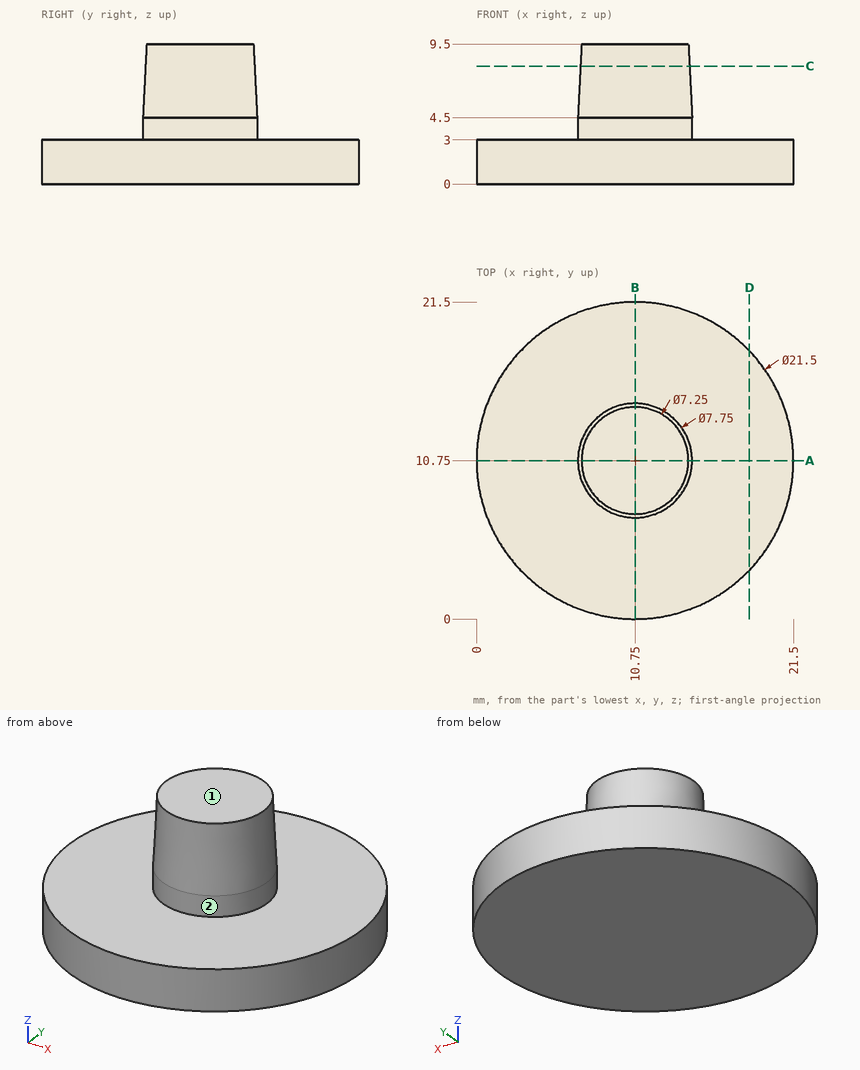
Could you check a few things on this drawing? It's one solid part, dimensions in mm from its lowest x, y, z. A direction names the side the tool comes from. Give positions to 0.01 mm unless a question says otherwise; leave off trailing zeros. Write each loop counter-clockwise with the first axis right and the second up, starting at its lowest first coordinate (ties: lowest second). Pieces come first, ordered by that corner, then holes. Notation, with made-up numbers: M 59.25,89 L 106.25,89 A13 cw 106.25,112 Z; hole C 12.5,83 d3. An arc over 180 degrees is marked long. Put each result on its own line as item: value. Start each with the question number.
Item 1: I need wall thicknesses on L1, parallel to Z at x = 9.25, y = 19; L2, parallel to X at y = 13, z = 1; L3, parallel to X at y = 8, z = 4.25. Which ranges of each line are inside material? Lowest first, please. Write a range as from..to.
Item 2: If we section it at A-A, the plane y = 10.75: Write out the boundary of the cut face in (x, z) (3 decimals).
Item 3: Will these pins go through, and if not, where does the flat tip stop? pin 1 (4 mm diameter, centred on x = 3, z = 4.5, fed in from +Y); pin 2 (1 mm diameter, centred on x = 7, z = 7.5, fed in from -Y); pin 3 (5 mm diameter, centred on x = 11, z = 6.5, fed in from -Y) (3 decimals).
Item 4: If we section it at C-C, the plane z = 8: Write out the boundary of the cut face in (x, y).
Item 5: If we section it at D-D, the plane x = 18.5: Write out the boundary of the cut face in (y, z).
Item 6: On a 3-axis mill with a long thin cutter (end or side, diameter ignored), from which of +Z, -Z, +X, -X, +Y, -Y can I reach the whole of each face in a straight line? I mean the marked faces 1 and 2. Say none if no direction works.
Values:
1. L1: 0..3
1. L2: 0.24..21.26
1. L3: 8.02..13.48
2. outline: M 0,0 L 21.5,0 L 21.5,3 L 14.625,3 L 14.625,4.5 L 14.375,9.5 L 7.125,9.5 L 6.875,4.5 L 6.875,3 L 0,3 Z
3. pin 1: y = 19.37
3. pin 2: y = 8.93
3. pin 3: y = 6.875
4. outline: C 10.75,10.75 d7.4
5. outline: M 3.3,0 L 18.2,0 L 18.2,3 L 3.3,3 Z
6. face 1: +Z, +X, -X, +Y, -Y
6. face 2: +Z
